from build123d import *

# Parameters (mm, degrees)
F1_DEPTH       = 6.35
F2_DEPTH       = 12.7
F4_D           = 17.78
F4_CBORE_D     = 22.86
F4_CBORE_DEPTH = 6.35


with BuildPart() as f1:
    # F0 (on Top) → F1 (new body)
    with BuildSketch(Plane.XY):
        Polygon((50.8, 76.2), (-50.8, 76.2), (-50.8, -76.2), (50.8, -76.2), (50.8, 0), align=None)
        Polygon((48.26, 12.7), (48.26, 0), (48.26, -12.7), (22.86, -12.7), (22.86, 12.7), align=None, mode=Mode.SUBTRACT)
    extrude(amount=F1_DEPTH)

    # F0 (on Top) → F2 (join)
    with BuildSketch(Plane.XY):
        Polygon((48.26, -12.7), (48.26, 0), (48.26, 12.7), (22.86, 12.7), (22.86, -12.7), align=None)
    extrude(amount=F2_DEPTH)

    # F4 (through all)
    with Locations(Plane.XY.offset(12.7)):
        with Locations((35.56, 0)):
            CounterBoreHole(F4_D / 2, F4_CBORE_D / 2, F4_CBORE_DEPTH)


solid = f1.part
Build history of the part. All positions in model axes, mm. A direction names the side the tool comes from. Round coordinates to 2 decimals unless told otherwise and drop trailing zeros. Write each loop counter-clockwise with the first axis right and the second up, starting at its lowest first coordinate (ties: lowest second). Pieces come first, ordered by that corner, then holes. Notation, with made-up numbers: (24, -29.75) - (45, -29.75) arc R16 ccw to (45, -0.75) - close; hole circle Ø11 at (18.5, 78.25). An arc over 180 degrees is marked (long way). Use CSV: the item, a comma, the result in double quotes.
(1) Wall check: line 1 (Z direction, x = -21, y = 53); line 2 (Y direction, x = 35.56, z = 9.5); line 3 (X direction, y = 2, z = 10.25). Give the ranges that are in metal, low to high.
Response:
line 1,"0 to 6.35"
line 2,"-12.7 to -11.43, 11.43 to 12.7"
line 3,"22.86 to 24.31, 46.81 to 48.26"
(2) Band-saw the part on D-D (x = -13). Write the cut outline in (y, z), plus the area to 3 significant figures.
Response:
outline,"(-76.2, 0) - (76.2, 0) - (76.2, 6.35) - (-76.2, 6.35) - close"
area,"968 mm²"
(3) Band-saw the part on C-C (z = 8.5). Write the cut outline in (x, y), plus the area to 3 significant figures.
Response:
outline,"(22.86, -12.7) - (48.26, -12.7) - (48.26, 12.7) - (22.86, 12.7) - close; hole circle Ø22.86 at (35.56, 0)"
area,"235 mm²"
(4) Band-saw the part on A-A (y = 0). Write the cut outline in (x, z), plus the area to 3 significant figures.
Response:
outline,"(-50.8, 0) - (26.67, 0) - (26.67, 6.35) - (24.13, 6.35) - (24.13, 12.7) - (22.86, 12.7) - (22.86, 6.35) - (-50.8, 6.35) - close; (44.45, 0) - (50.8, 0) - (50.8, 6.35) - (48.26, 6.35) - (48.26, 12.7) - (46.99, 12.7) - (46.99, 6.35) - (44.45, 6.35) - close"
area,"548 mm²"
(5) Band-saw the part on B-B (x = 35.56). Write the cut outline in (y, z), plus the area to 3 significant figures.
Response:
outline,"(-76.2, 0) - (-8.89, 0) - (-8.89, 6.35) - (-11.43, 6.35) - (-11.43, 12.7) - (-12.7, 12.7) - (-12.7, 6.35) - (-76.2, 6.35) - close; (8.89, 0) - (76.2, 0) - (76.2, 6.35) - (12.7, 6.35) - (12.7, 12.7) - (11.43, 12.7) - (11.43, 6.35) - (8.89, 6.35) - close"
area,"871 mm²"
(6) Pin check, flat tips, straight feed: P1, Ø1.9, axis at y = 1.5, z = 9.5, coming from the +X side; P2, Ø5, axis at x = 35, z = 10, coming from the -Y side; P3, Ø5, axis at x = 21.5, y = 36.5, coming from the +Z side. Stop position of each tip, or through.
Response:
P1,"x = 48.26"
P2,"y = -12.7"
P3,"z = 6.35"
(7) Mould opens along Y. For faces 1 (the flat face through (35, -12.7, 9)), 2 (the flat face through (28.7, -5.9, 6.35)), 3 (the flat face through (-1, 1, 0)), 4 (the cylindrical face through (24.14, 0.5, 9.57)) say: pulls with the +Y half, pulls with the -Y half, needs draft (parallel to the pull), parting line crosses it, or undercut.
Response:
face 1,"pulls with the -Y half"
face 2,"undercut"
face 3,"needs draft"
face 4,"undercut"
(8) 3-axis set-ups, long thin cutter, end or side, ignore diameter. For faces 5 (the flat face through (48.26, 0, 9)), 6 (the flat face through (22.86, 0, 9)), 7 (the flat face through (50.8, -1, 3)), 8 (the flat face through (36, 12.7, 9)): which of +Z, -Z, +X, -X, +Y, -Y reach the whole face in a straight line?
Response:
face 5,"+Z, +X, +Y, -Y"
face 6,"+Z, -X, +Y, -Y"
face 7,"+Z, -Z, +X, +Y, -Y"
face 8,"+Z, +X, -X, +Y"
